Could you check a few things on this model? Use its own coordinates, in mm. A direction names the side the tool comes from. Give positions to 0.01 mm unless a question says otherwise; leave off trailing zeros. Order: outer loops, then holes, each group sorted by start corner. A loop starts at its lowest first (then second) coordinate and runs counter-clockwise, first axis right, second up.
from build123d import *

# Parameters (mm, degrees)
F2_W     = 25
F2_H     = 10
F3_DEPTH = 60
F5_DEPTH = 12.5
F8_DEPTH = 60


with BuildPart() as f3:
    # F2 (on Top) → F3 (new body)
    with BuildSketch(Plane.XY):
        with Locations((0, 5)):
            Rectangle(F2_W, F2_H)
    extrude(amount=F3_DEPTH)

    # F4 (on Right) → F5 (join, symmetric)
    with BuildSketch(Plane.YZ):
        Polygon((10, 60), (10, 0), (15.25, 60), align=None)
    extrude(amount=F5_DEPTH, both=True)

    # F7 (on face) → F8 (cut, through all)
    with BuildSketch(Plane.XY.offset(60)):
        Polygon((-9.5, 4), (-7.5, 0), (7.5, 0), (9.5, 4), align=None)
    extrude(amount=-F8_DEPTH, mode=Mode.SUBTRACT)


solid = f3.part
Item 1: Imagine slicing it at B-B on z = 48. List the corners of the cut face in (x, y) for me.
Findings:
outline: (-12.5, 0) - (-7.5, 0) - (-9.5, 4) - (9.5, 4) - (7.5, 0) - (12.5, 0) - (12.5, 14.2) - (-12.5, 14.2) - close
Item 2: We'd pull the mould along X, two halves only. Please class faces 3 (the flat face through (-12.5, 6, 30)), 4 (the flat face through (0.18, 12.59, 29.58)), 5 (the flat face through (-8.5, 2, 30.4)): +X half, -X half, draft (parallel to the pull), parting line (faces both ways), or undercut.
Findings:
face 3: -X half
face 4: draft
face 5: undercut
Item 3: Imagine slicing it at D-D on z = 40. List the corners of the cut face in (x, y) for me.
Findings:
outline: (-12.5, 0) - (-7.5, 0) - (-9.5, 4) - (9.5, 4) - (7.5, 0) - (12.5, 0) - (12.5, 13.5) - (-12.5, 13.5) - close
Item 4: Please list where these lines run through material, in increasing order: line 1 along X through (y, z) = (1, 55.5); line 2 along X through (y, z) = (3.75, 50) (3 decimals); line 3 along Y through (x, z) = (-9, 12).
Findings:
line 1: x = -12.5 to -8, 8 to 12.5
line 2: x = -12.5 to -9.375, 9.375 to 12.5
line 3: y = 0 to 3, 4 to 11.05
Item 5: Imagine slicing it at A-A on x = 8.5. List the corners of the cut face in (y, z) for me, then the cut area to 4 significant figures.
Findings:
outline: (0, 0) - (2, 0) - (2, 60) - (0, 60) - close; (4, 0) - (10, 0) - (15.25, 60) - (4, 60) - close
area: 637.5 mm2
Item 6: Imagine slicing it at C-C on x = -3.25. List the corners of the cut face in (y, z) for me, then the cut area to 4 significant figures.
Findings:
outline: (4, 0) - (10, 0) - (15.25, 60) - (4, 60) - close
area: 517.5 mm2
Item 7: For faces 1 (the flat face through (0, 9, 60)), 2 (the flat face through (0, 4, 30)), which set-ups out of +Z, -Z, +X, -X, +Y, -Y let a thin tool reach every point of the face, with its end or its side?
Findings:
face 1: +Z, +X, -X, +Y, -Y
face 2: +Z, -Z
Item 8: For pin 1 (10 mm diameter, centred on x = -3.5, z = 50.5, fed in from +Y); pin 2 (10 mm diameter, centred on x = -4.5, z = 12, fed in from +Y); pin 3 (4 mm diameter, centred on x = -3.5, z = 39.5, fed in from +Y), each with a flat end and sliding along its axis, tell me the tip position at first contact or that it passes through.
Findings:
pin 1: stops at y = 14.86
pin 2: stops at y = 11.49
pin 3: stops at y = 13.63
